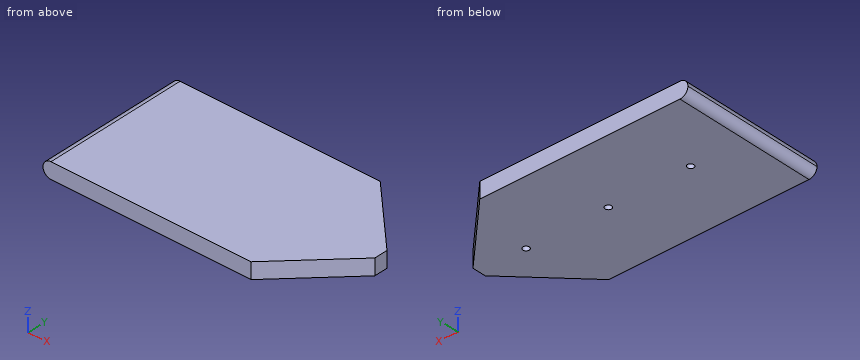
from build123d import *

# Parameters (mm, degrees)
F1_DEPTH    = 12.7
F2_D        = 5.08
F2_DEPTH    = 5.08
F2_TIP      = 1.5261859723
F3_D        = 5.08
F3_DEPTH    = 5.08
F3_TIP      = 1.5261859723
F4_T1_DEPTH = 339.3037394717
F5_SIZE     = 7.62
F6_R        = 6.34999


# Not quite as in the source:
# - a fillet or chamfer that OpenCascade refuses, or shapes differently, is made with other operations: its cross-section is extruded or revolved along the edge and cut away or added
# - a fillet or chamfer is up to 0.001 mm smaller than in the source, because OpenCascade refuses the exact size


with BuildPart() as f1:
    # F0 (on Top) → F1 (new body)
    with BuildSketch(Plane.XY):
        Polygon((114.3, 27.94), (114.3, 57.15), (82.55, 57.15), (-114.3, 57.15), (-114.3, -57.15), (82.55, -57.15), (114.3, -57.15), (114.3, -27.94), align=None)
    extrude(amount=F1_DEPTH)

    # F2
    with Locations(Plane(origin=(0, 0, 0), x_dir=(1, 0, 0), z_dir=(0, 0, -1))):
        with Locations((-65.25006, 0)):
            Hole(F2_D / 2, depth=F2_DEPTH)
            with Locations((0, 0, -(F2_DEPTH + F2_TIP / 2))):  # 118° drill point
                Cone(0, F2_D / 2, F2_TIP, mode=Mode.SUBTRACT)

    # F3
    with Locations(Plane(origin=(0, 0, 0), x_dir=(1, 0, 0), z_dir=(0, 0, -1))):
        with Locations((0, 0), (65.25006, 0)):
            Hole(F3_D / 2, depth=F3_DEPTH)
            with Locations((0, 0, -(F3_DEPTH + F3_TIP / 2))):  # 118° drill point
                Cone(0, F3_D / 2, F3_TIP, mode=Mode.SUBTRACT)

    # F4: chamfer of 63.5 on 2 edges, made by hand

    # F4_s2 → F4_t1 (cut)
    with BuildSketch(Plane.XY.offset(-163.3018697358)):
        Polygon((114.3, -6.35), (50.8, 57.15), (114.3, 57.15), align=None)
        Polygon((114.3, 6.35), (50.8, -57.15), (114.3, -57.15), align=None)
    extrude(amount=F4_T1_DEPTH, mode=Mode.SUBTRACT)

    # F5
    f5_edges = [f1.edges().sort_by_distance(p)[0] for p in [
        (107.95, 0, 6.35),
    ]]
    chamfer(f5_edges, length=F5_SIZE)

    # F6 (radius 6.35 in the source; OpenCascade refuses exactly that, so slightly less here)
    f6_edges = [f1.edges().sort_by_distance(p)[0] for p in [
        (-114.3, 0, 0),
        (-114.3, 0, 12.7),
    ]]
    fillet(f6_edges, radius=F6_R)


solid = f1.part
Read the model definition and answer for the solid it produces. Units are mm, in the model's axes. Give positions to 0.01 mm unless a question says otherwise; leave off trailing zeros. Write each loop counter-clockwise with the first axis right and the second up, starting at its lowest first coordinate (ties: lowest second). Pieces come first, ordered by that corner, then holes. Notation, with made-up numbers: (64, 55.5) - (72, 55.5) arc R32 cw to (72, 87.5) - close; hole circle Ø5 at (10.5, 66). An arc over 180 degrees is marked (long way). Use CSV: the item, a comma, the result in double quotes. Start each with the question number.
Item 1: A flat-ended cylindrical pin translates along its axis: P1, Ø4, axis at y = -19.5, z = 5, coming from the +X side. Find the tip coordinate at first contact, or state that the pin passes through.
Item 2: The part is cut by section C-C, the plane x = 86.5. Give the vertices of the cut face in (y, z), and give its area (3 significant figures).
Item 3: Consider line 1 (Y direction, x = 0, z = 3.2); line 2 (X direction, y = -31.5, z = 7.5) (3 decimals); line 3 (X direction, y = 6.5, z = 6). Determine where each line is inside the solid, lowest interval first.
Item 4: The part is cut by section B-B, the plane z = 2. Give the vertices of the cut face in (x, y), and give its area (3 significant figures).
Taken from the geometry:
1,P1,"x = 90.45"
2,outline,"(-21.45, 0) - (21.45, 0) - (21.45, 12.7) - (-21.45, 12.7) - close"
2,area,"545 mm2"
3,line 1,"-57.15 to -2.54, 2.54 to 57.15"
3,line 2,"-114.195 to 76.45"
3,line 3,"-114.29 to 101.45"
4,outline,"(-112.58, -57.15) - (50.8, -57.15) - (102.56, -5.39) - (102.56, 5.39) - (50.8, 57.15) - (-112.58, 57.15) - close; hole circle Ø5.08 at (-65.25, 0); hole circle Ø5.08 at (0, 0); hole circle Ø5.08 at (65.25, 0)"
4,area,"21,900 mm2"
